Work out the finished part from the listing and answer in its coordinate system (mm). A direction names the side the tool comes from. Round coordinates to 2 decimals unless told otherwise and drop trailing zeros. Loops run counter-clockwise (first coordinate to the right, second up) from the corner with the lowest first, then second, coordinate; pieces in that order, holes last. Notation, with made-up numbers: M 57,38.5 L 116,38.5 A13 cw 116,60.5 Z; hole C 22.25,86.5 d1. An arc over 180 degrees is marked long. One line per item, written item: value.
```python
from build123d import *

# Parameters (mm, degrees)
RESSALTO_EXTRUS_O1_DEPTH = 30
ESBO_O2_W                = 12
ESBO_O2_H                = 94
CORTE_EXTRUS_O1_DEPTH    = 118.541482039
ESBO_O3_W                = 30
ESBO_O3_H                = 10
CORTE_EXTRUS_O2_DEPTH    = 118.541482039
ESBO_O4_W                = 3.6
ESBO_O4_H                = 30
CORTE_EXTRUS_O3_DEPTH    = 108.498837203
ESBO_O5_W                = 56.4
ESBO_O5_H                = 6
RESSALTO_EXTRUS_O2_DEPTH = 16
ESBO_O6_W                = 56.4
ESBO_O6_H                = 6
RESSALTO_EXTRUS_O3_DEPTH = 16
FILETE1_R                = 8
FILETE2_R                = 8
FILETE3_R                = 8
FILETE4_R                = 4
ESBO_O7_R                = 3.175
CORTE_EXTRUS_O4_DEPTH    = 113.943171551
ESBO_O8_R                = 3.25
CORTE_EXTRUS_O5_DEPTH    = 112.143870726
ESBO_O9_W                = 56.4
ESBO_O9_H                = 62
CORTE_EXTRUS_O6_DEPTH    = 112.143870726
ESBO_O10_W               = 26.4
ESBO_O10_H               = 4.76
CORTE_EXTRUS_O7_DEPTH    = 74.027118251
ESBO_O11_W               = 4.76
ESBO_O11_H               = 62
CORTE_EXTRUS_O8_DEPTH    = 74.027118251


with BuildPart() as part:
    # Esboço1 → Ressalto-extrusão1 (new body)
    with BuildSketch(Plane.XY):
        Polygon((0, 0), (0, 100), (60, 0), align=None)
    extrude(amount=RESSALTO_EXTRUS_O1_DEPTH)

    # Esboço2 → Corte-extrusão1 (cut, through all)
    with BuildSketch(Plane.ZY.offset(-6)):
        with Locations((24, 53)):
            Rectangle(ESBO_O2_W, ESBO_O2_H)
        with Locations((6, 53)):
            Rectangle(ESBO_O2_W, ESBO_O2_H)
    extrude(amount=-CORTE_EXTRUS_O1_DEPTH, mode=Mode.SUBTRACT)

    # Esboço3 → Corte-extrusão2 (cut, through all)
    with BuildSketch(Plane(origin=(6, 0, 0), x_dir=(0, 0, -1), z_dir=(1, 0, 0))):
        with Locations((-15, 95)):
            Rectangle(ESBO_O3_W, ESBO_O3_H)
    extrude(amount=-CORTE_EXTRUS_O2_DEPTH, mode=Mode.SUBTRACT)

    # Esboço4 → Corte-extrusão3 (cut, through all)
    with BuildSketch(Plane(origin=(0, 6, 0), x_dir=(1, 0, 0), z_dir=(0, 1, 0))):
        with Locations((58.2, -15)):
            Rectangle(ESBO_O4_W, ESBO_O4_H)
    extrude(amount=-CORTE_EXTRUS_O3_DEPTH, mode=Mode.SUBTRACT)

    # Esboço5 → Ressalto-extrusão2 (add)
    with BuildSketch(Plane.XY.offset(30)):
        with Locations((28.2, 3)):
            Rectangle(ESBO_O5_W, ESBO_O5_H)
    extrude(amount=RESSALTO_EXTRUS_O2_DEPTH)

    # Esboço6 → Ressalto-extrusão3 (add)
    with BuildSketch(Plane(origin=(0, 0, 0), x_dir=(-1, 0, 0), z_dir=(0, 0, -1))):
        with Locations((-28.2, 3)):
            Rectangle(ESBO_O6_W, ESBO_O6_H)
    extrude(amount=RESSALTO_EXTRUS_O3_DEPTH)

    # Filete1
    filete1_edges = [part.edges().sort_by_distance(p)[0] for p in [
        (3, 6, 0),
        (3, 6, 30),
    ]]
    fillet(filete1_edges, radius=FILETE1_R)

    # Filete2
    filete2_edges = [part.edges().sort_by_distance(p)[0] for p in [
        (56.4, 3, -16),
        (56.4, 3, 46),
    ]]
    fillet(filete2_edges, radius=FILETE2_R)

    # Filete3
    filete3_edges = [part.edges().sort_by_distance(p)[0] for p in [
        (3, 90, 30),
        (3, 90, 0),
    ]]
    fillet(filete3_edges, radius=FILETE3_R)

    # Filete4
    filete4_edges = [part.edges().sort_by_distance(p)[0] for p in [
        (31.2, 6, 18),
        (31.2, 6, 12),
    ]]
    fillet(filete4_edges, radius=FILETE4_R)

    # Esboço7 → Corte-extrusão4 (cut, through all)
    with BuildSketch(Plane(origin=(6, 0, 0), x_dir=(0, 0, -1), z_dir=(1, 0, 0))):
        with Locations((-23, 78)):
            Circle(ESBO_O7_R)
        with Locations((-23, 48)):
            Circle(ESBO_O7_R)
        with Locations((-23, 18)):
            Circle(ESBO_O7_R)
        with Locations(Location((-7, 18, 0), (0, 0, 180))):
            Circle(ESBO_O7_R)
        with Locations(Location((-7, 48, 0), (0, 0, 180))):
            Circle(ESBO_O7_R)
        with Locations(Location((-7, 78, 0), (0, 0, 180))):
            Circle(ESBO_O7_R)
    extrude(amount=-CORTE_EXTRUS_O4_DEPTH, mode=Mode.SUBTRACT)

    # Esboço8 → Corte-extrusão5 (cut, through all)
    with BuildSketch(Plane(origin=(0, 6, 0), x_dir=(1, 0, 0), z_dir=(0, 1, 0))):
        with Locations(Location((48.4, 8, 0), (0, 0, 270))):
            Circle(ESBO_O8_R)
        with Locations(Location((48.4, -38, 0), (0, 0, 270))):
            Circle(ESBO_O8_R)
        with Locations(Location((16.4, -38, 0), (0, 0, 270))):
            Circle(ESBO_O8_R)
        with Locations(Location((16.4, 8, 0), (0, 0, 270))):
            Circle(ESBO_O8_R)
    extrude(amount=-CORTE_EXTRUS_O5_DEPTH, mode=Mode.SUBTRACT)

    # Esboço9 → Corte-extrusão6 (cut, through all)
    with BuildSketch(Plane(origin=(0, 6, 0), x_dir=(1, 0, 0), z_dir=(0, 1, 0))):
        with Locations((28.2, -15)):
            Rectangle(ESBO_O9_W, ESBO_O9_H)
    extrude(amount=CORTE_EXTRUS_O6_DEPTH, mode=Mode.SUBTRACT)

    # Esboço10 → Corte-extrusão7 (cut, through all)
    with BuildSketch(Plane(origin=(0, 6, 0), x_dir=(1, 0, 0), z_dir=(0, 1, 0))):
        with Locations((28.2, -15)):
            Rectangle(ESBO_O10_W, ESBO_O10_H)
    extrude(amount=-CORTE_EXTRUS_O7_DEPTH, mode=Mode.SUBTRACT)

    # Esboço11 → Corte-extrusão8 (cut, through all)
    with BuildSketch(Plane(origin=(0, 6, 0), x_dir=(1, 0, 0), z_dir=(0, 1, 0))):
        with Locations((2.38, -15)):
            Rectangle(ESBO_O11_W, ESBO_O11_H)
    extrude(amount=-CORTE_EXTRUS_O8_DEPTH, mode=Mode.SUBTRACT)


solid = part.part
```
1) Find section C-C (y = 4.4). Give the vertices of the cut face in (x, z), then the cut area to 3 significant figures.
Check values:
outline: M 4.76,-16 L 48.4,-16 A8 ccw 56.4,-8 L 56.4,38 A8 ccw 48.4,46 L 4.76,46 Z; hole C 16.4,-8 d6.5; hole C 16.4,38 d6.5; hole M 15,12.62 L 41.4,12.62 L 41.4,17.38 L 15,17.38 Z; hole C 48.4,-8 d6.5; hole C 48.4,38 d6.5
area: 2,920 mm2
2) Find section B-B (x = 23). Give the vertices of the cut face in (y, z), then the cut area to 3 significant figures.
Check values:
outline: M 0,-16 L 6,-16 L 6,12.62 L 0,12.62 Z; M 0,17.38 L 6,17.38 L 6,46 L 0,46 Z
area: 343 mm2
3) The mould has two halves that part along X. Classify faces 3 (the face through (31, 6, 22)), 4 (the face through (28, 3, 12.62)), 5 (the face through (56.4, 3, 15)): +X half, -X half, draft (parallel to the pull), parting line (faces both ways), or undercut.
Check values:
face 3: draft
face 4: undercut
face 5: +X half
4) Find section D-D (z = 42). Give the vertices of the cut face in (x, y), then the cut area to 3 significant figures.
Check values:
outline: M 4.76,0 L 55.33,0 L 55.33,6 L 4.76,6 Z
area: 303 mm2
5) Find the intervals of material crossed by probe 1 along X at (y, z) = (2.9, -8); probe 2 along X at (y, z) = (5.6, 13); probe 3 along Z at (x, y) = (48, 0.4), in increasing order. Write a range as from..to.
Check values:
probe 1: 4.76..13.15, 19.65..45.15, 51.65..56.4
probe 2: 4.76..15, 41.4..56.4
probe 3: -16..-11.23, -4.77..34.77, 41.23..46
6) Find section A-A (x = 16.4). Give the vertices of the cut face in (y, z), then the cut area to 3 significant figures.
Check values:
outline: M 0,-16 L 6,-16 L 6,-11.25 L 0,-11.25 Z; M 0,-4.75 L 6,-4.75 L 6,12.62 L 0,12.62 Z; M 0,17.38 L 6,17.38 L 6,34.75 L 0,34.75 Z; M 0,41.25 L 6,41.25 L 6,46 L 0,46 Z
area: 265 mm2
7) For faces 1 (the face through (27, 3, -16)), 2 (the face through (41.4, 3, 15)), determine the directions among +Z, -Z, +X, -X, +Y, -Y from which every point of the face is accessible in a straight line to the end or side of a thin tool.
Check values:
face 1: -Z, +X, -X, +Y, -Y
face 2: +Y, -Y
